CAD build for the part. Positions are in the model's coordinates, mm. A direction names the side the tool comes from. Give positions to 0.01 mm unless a question says otherwise; leave off trailing zeros. Loops run counter-clockwise (first coordinate to the right, second up) from the corner with the lowest first, then second, coordinate; pieces in that order, holes last. Notation, with made-up numbers: (50, -12) - (63, -12) arc R9 cw to (63, 3) - close; hole circle Ø2 at (60.25, 19). An arc over 180 degrees is marked (long way). Return JSON: item names as keys, results as strings.
from build123d import *

# Parameters (mm, degrees)
SKETCH1_W           = 76.2
SKETCH1_H           = 25.4
SKETCH1_W_2         = 69.85
SKETCH1_H_2         = 19.05
BOSS_EXTRUDE1_DEPTH = 177.8
SKETCH4_R           = 3.3782
CUT_EXTRUDE1_DEPTH  = 26.4
SKETCH5_R           = 3.3782
CUT_EXTRUDE2_DEPTH  = 26.4
SKETCH6_R           = 3.3782
CUT_EXTRUDE3_DEPTH  = 26.4
SKETCH7_R           = 5.0419
CUT_EXTRUDE4_DEPTH  = 26.4


with BuildPart() as part:
    # Sketch1 → Boss-Extrude1 (new body)
    with BuildSketch(Plane.XY):
        with Locations((38.1, 12.7)):
            Rectangle(SKETCH1_W, SKETCH1_H)
        with Locations((38.1, 12.7)):
            Rectangle(SKETCH1_W_2, SKETCH1_H_2, mode=Mode.SUBTRACT)
    extrude(amount=BOSS_EXTRUDE1_DEPTH)

    # Sketch4 → Cut-Extrude1 (cut, through all)
    with BuildSketch(Plane(origin=(0, 25.4, 0), x_dir=(1, 0, 0), z_dir=(0, 1, 0))):
        with Locations((13.21308, -16.2687)):
            Circle(SKETCH4_R)
        with Locations((29.80436, -16.2687)):
            Circle(SKETCH4_R)
        with Locations((46.39564, -16.2687)):
            Circle(SKETCH4_R)
        with Locations((62.98692, -16.2687)):
            Circle(SKETCH4_R)
    extrude(amount=-CUT_EXTRUDE1_DEPTH, mode=Mode.SUBTRACT)

    # Sketch5 → Cut-Extrude2 (cut, through all)
    with BuildSketch(Plane.XZ):
        with Locations((12.7, 167.819500474)):
            Circle(SKETCH5_R)
    extrude(amount=-CUT_EXTRUDE2_DEPTH, mode=Mode.SUBTRACT)

    # Sketch6 → Cut-Extrude3 (cut, through all)
    with BuildSketch(Plane(origin=(0, 25.4, 0), x_dir=(1, 0, 0), z_dir=(0, 1, 0))):
        with Locations((63.5, -161.5313)):
            Circle(SKETCH6_R)
        with Locations((34.925, -161.5313)):
            Circle(SKETCH6_R)
    extrude(amount=-CUT_EXTRUDE3_DEPTH, mode=Mode.SUBTRACT)

    # Sketch7 → Cut-Extrude4 (cut, through all)
    with BuildSketch(Plane.XZ):
        with Locations((15.875, 12.7)):
            Circle(SKETCH7_R)
        with Locations((60.325, 12.7)):
            Circle(SKETCH7_R)
    extrude(amount=-CUT_EXTRUDE4_DEPTH, mode=Mode.SUBTRACT)


solid = part.part
1. Cut at B-B, the plane z = 131.5. Write the cut outline in (x, y) (3 decimals).
Values follow:
{"outline": "(0, 0) - (76.2, 0) - (76.2, 25.4) - (0, 25.4) - close; hole (3.175, 3.175) - (73.025, 3.175) - (73.025, 22.225) - (3.175, 22.225) - close"}
2. Pull direction Z, two halves, no side cores. Call faces 1 (the face through (76.2, 13, 88)), 2 (the face through (63.06, 1.61, 158.18)), 3 (the face through (35, 2, 177.8)), 4 (the face through (35, 2, 0)): +Z half, -Z half, draft (parallel to the pull), parting line (faces both ways), or undercut.
Values follow:
{"face 1": "draft", "face 2": "undercut", "face 3": "+Z half", "face 4": "-Z half"}
3. Drop flat-ended pins along their axis: P1, Ø3, axis at x = 66.5, y = 22, coming from the -Z side; P2, Ø2, axis at x = 37.5, y = 6, coming from the +Z side. Give the stop position or say it passes through.
Values follow:
{"P1": "stops at z = 0", "P2": "passes through"}
4. Cut at C-C, the plane x = 47.5. Write the cut outline in (y, z) (3 decimals).
Values follow:
{"outline": "(0, 0) - (3.175, 0) - (3.175, 13.076) - (0, 13.076) - close; (0, 19.461) - (3.175, 19.461) - (3.175, 177.8) - (0, 177.8) - close; (22.225, 0) - (25.4, 0) - (25.4, 13.076) - (22.225, 13.076) - close; (22.225, 19.461) - (25.4, 19.461) - (25.4, 177.8) - (22.225, 177.8) - close"}
5. Cut at A-A, the plane y = 18.25. Write the cut outline in (x, z) (3 decimals), plus the area to 3 significant figures.
Values follow:
{"outline": "(0, 0) - (3.175, 0) - (3.175, 177.8) - (0, 177.8) - close; (73.025, 0) - (76.2, 0) - (76.2, 177.8) - (73.025, 177.8) - close", "area": "1,130 mm²"}
6. Drill centre lines: probe 1 along X at (y, z) = (7.5, 154) (3 decimals); probe 2 along Y at (x, z) = (7, 67) (3 decimals); probe 3 along Z at (x, y) = (63.5, 1.45). Where is each one in solid material? Low to high.
Values follow:
{"probe 1": "x = 0 to 3.175, 73.025 to 76.2", "probe 2": "y = 0 to 3.175, 22.225 to 25.4", "probe 3": "z = 0 to 8.78, 19.61 to 158.15, 164.91 to 177.8"}
7. Cut at D-D, the plane x = 12.7. Write the cut outline in (y, z) (3 decimals), plus the area to 3 significant figures.
Values follow:
{"outline": "(0, 0) - (3.175, 0) - (3.175, 8.783) - (0, 8.783) - close; (0, 19.608) - (3.175, 19.608) - (3.175, 164.441) - (0, 164.441) - close; (0, 171.198) - (3.175, 171.198) - (3.175, 177.8) - (0, 177.8) - close; (22.225, 0) - (25.4, 0) - (25.4, 8.783) - (22.225, 8.783) - close; (22.225, 19.608) - (25.4, 19.608) - (25.4, 164.441) - (22.225, 164.441) - close; (22.225, 171.198) - (25.4, 171.198) - (25.4, 177.8) - (22.225, 177.8) - close", "area": "1,020 mm²"}
8. Which spindle directions (+Z, -Z, +X, -X, +Y, -Y) get a long thin tool onto all of the face, cutting with end or side? Do faces 5 (the face through (3.175, 13, 88)), 6 (the face through (12.26, 23.79, 171.17)). Say none if no direction does.
Values follow:
{"face 5": "+Z, -Z", "face 6": "+Y, -Y"}
